```python
from build123d import *

# Parameters (mm, degrees)
SKETCH_1_W          = 145
SKETCH_1_H          = 54.239140964
SKETCH_1_R          = 15
EXTRUDE_1_DEPTH     = 14
SKETCH_2_W          = 40.973545211
SKETCH_2_H          = 20
CUT_EXTRUDE_1_DEPTH = 50
SKETCH_3_R          = 2.5
CUT_EXTRUDE_2_DEPTH = 36
SKETCH_4_W          = 40.34248958
SKETCH_4_H          = 54.239140964
SKETCH_4_R          = 15
EXTRUDE_2_DEPTH     = 16


with BuildPart() as part:
    # Эскиз1 → Вытянуть1 (new body)
    with BuildSketch(Plane(origin=(0, 0, 0), x_dir=(1, 0, 0), z_dir=(0, 1, 0))):
        with Locations((52.5, 0)):
            Rectangle(SKETCH_1_W, SKETCH_1_H)
        with Locations(Location((0, 0, 0), (0, 0, 270))):
            Circle(SKETCH_1_R, mode=Mode.SUBTRACT)
    extrude(amount=EXTRUDE_1_DEPTH)

    # Эскиз2 → Вырез-Вытянуть1 (cut)
    with BuildSketch(Plane(origin=(0, 0, 0), x_dir=(1, 0, 0), z_dir=(0, 1, 0))):
        with Locations((110.055787262, 0)):
            Rectangle(SKETCH_2_W, SKETCH_2_H)
    extrude(amount=CUT_EXTRUDE_1_DEPTH, mode=Mode.SUBTRACT)

    # Эскиз3 → Вырез-Вытянуть2 (cut, symmetric)
    with BuildSketch(Plane.XY):
        with Locations(Location((107.871367235, 7.461129595, 0), (0, 0, 180))):
            Circle(SKETCH_3_R)
    extrude(amount=CUT_EXTRUDE_2_DEPTH, both=True, mode=Mode.SUBTRACT)

    # Эскиз4 → Вытянуть2 (add)
    with BuildSketch(Plane(origin=(0, 14, 0), x_dir=(1, 0, 0), z_dir=(0, 1, 0))):
        with Locations((0.17124479, 0)):
            Rectangle(SKETCH_4_W, SKETCH_4_H)
        with Locations(Location((0, 0, 0), (0, 0, 270))):
            Circle(SKETCH_4_R, mode=Mode.SUBTRACT)
    extrude(amount=EXTRUDE_2_DEPTH)


solid = part.part
```
Could you check a few things on this model? Use its own coordinates, in mm. A direction names the side the tool comes from. Round coordinates to 2 decimals unless told otherwise and drop trailing zeros. Loops run counter-clockwise (first coordinate to the right, second up) from the corner with the lowest first, then second, coordinate; pieces in that order, holes last. Notation, with made-up numbers: (-34.5, 17.25) -> (19.5, 17.25) arc R6 ccw to (19.5, 28.25) -> close; hole circle Ø2 at (85, 56). An arc over 180 degrees is marked (long way). One line per question, with ' | ' between items.
(1) Thinking about a two-plate mould opening in Z: for faces 1 (the face through (105.487, 6.71, 18.68)), 2 (the face through (107, 10, -10)), 3 (the face through (35, 11, -27.12)), which applies, released by +Z, released by -Z, zero draft, split by the parting line, or undercut?
Model answer:
face 1: zero draft | face 2: undercut | face 3: released by -Z
(2) If we section it at C-C on y = 16.75: List the corners of the cut face in (x, z) for me, and give its area (3 significant figures).
Model answer:
outline: (-20, -27.12) -> (20.34, -27.12) -> (20.34, 27.12) -> (-20, 27.12) -> close; hole circle Ø30 at (0, 0) | area: 1,480 mm^2
(3) If we section it at A-A on z = 12.5: List the corners of the cut face in (x, y) for me.
Model answer:
outline: (-20, 0) -> (-8.29, 0) -> (-8.29, 30) -> (-20, 30) -> close; (8.29, 0) -> (125, 0) -> (125, 14) -> (20.34, 14) -> (20.34, 30) -> (8.29, 30) -> close; hole circle Ø5 at (107.87, 7.46)
(4) If we section it at D-D on z = 0: List the corners of the cut face in (x, y) for me, and give its area (3 significant figures).
Model answer:
outline: (-20, 0) -> (-15, 0) -> (-15, 30) -> (-20, 30) -> close; (15, 0) -> (89.57, 0) -> (89.57, 14) -> (20.34, 14) -> (20.34, 30) -> (15, 30) -> close | area: 1,280 mm^2
(5) For pin 1 Ø5 at (y, z) = (26, -4) entering from +X; pin 2 Ø11 at (y, z) = (7.5, 0) entering from +X; pin 3 Ø12 at (x, z) = (54.5, -18) entering from +Y, each with a flat end and sliding along its axis, tell me the tip position at first contact or that it passes through.
Model answer:
pin 1: stops at x = 20.34 | pin 2: stops at x = 89.57 | pin 3: stops at y = 14
(6) If I drill on probe 1 along X at (y, z) = (13.75, 0); probe 2 along X at (y, z) = (15.25, 0); probe 3 along Y at (x, z) = (112, -11), over which ranges is the centre line in solid material (lowest first)?
Model answer:
probe 1: x = -20 to -15, 15 to 89.57 | probe 2: x = -20 to -15, 15 to 20.34 | probe 3: y = 0 to 14
(7) If we section it at B-B on x = 0: List the corners of the cut face in (y, z) for me, and give its area (3 significant figures).
Model answer:
outline: (0, -27.12) -> (30, -27.12) -> (30, -15) -> (0, -15) -> close; (0, 15) -> (30, 15) -> (30, 27.12) -> (0, 27.12) -> close | area: 727 mm^2
(8) For faces 4 (the face through (72, 14, 0)), 5 (the face through (105.487, 6.71, -18.44)), 6 (the face through (107, 10, 10)), which set-ups out of +Z, -Z, +X, -X, +Y, -Y let a thin tool reach every point of the face, with its end or its side?
Model answer:
face 4: +Z, -Z, +X, +Y | face 5: +Z, -Z | face 6: +X, +Y, -Y
